from build123d import *

# Parameters (mm, degrees)
F0_R     = 5
F1_DEPTH = 10


with BuildPart() as f1:
    # F0 (on Right) → F1 (new body)
    with BuildSketch(Plane.YZ):
        Polygon((223.333333, 94.888889), (223.333333, 194.888889), (-196.666667, 194.888889), (-196.666667, -355.111111), (-96.666667, -355.111111), (-96.666667, 94.888889), align=None)
        with Locations((-116.666667, 144.888889)):
            Circle(F0_R, mode=Mode.SUBTRACT)
        with Locations((183.333333, 144.888889)):
            Circle(F0_R, mode=Mode.SUBTRACT)
    extrude(amount=F1_DEPTH)


solid = f1.part
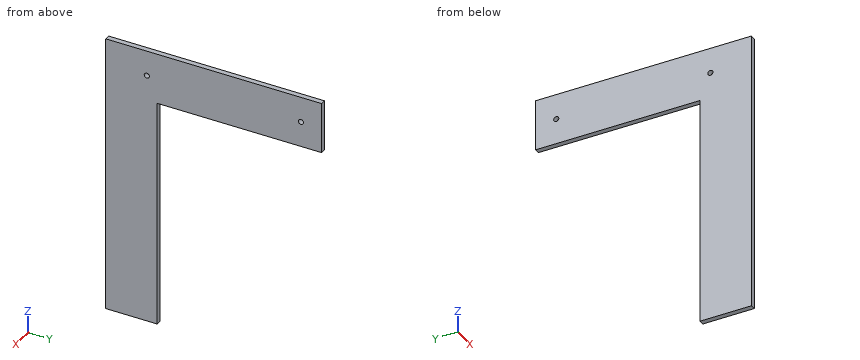
Geometry check sheet. Reference: the model listing, model coordinates, mm. Coordinates: 2 decimals unless noted, no trailing zeros. Order: outer loops, then holes, each group sorted by start corner. A loop starts at its lowest first (then second) coordinate and runs counter-clockwise, first axis right, second up. Notation, with made-up numbers: (-11.75, 16) -> (42.25, 16) arc R29 ccw to (42.25, 52) -> close; hole circle Ø1 at (75.5, -5). An arc over 180 degrees is marked (long way). Use a Markdown table: item, result. Add a question column.
1. Material ranges on L1, parallel to Y at x = 2, z = -186; L2, parallel to Z at x = 8.5, y = 73; L3, parallel to Z at x = 3.25, y = 184, recorded low to high.
2. Go/stop test with flat-tipped pins: pin 1 Ø2 at (x, y) = (2.5, 114) entering from -Z; pin 2 Ø1 at (y, z) = (-97.5, 44) entering from -X; pin 3 Ø9 at (y, z) = (183.33, 144.89) entering from +X; pin 4 Ø5 at (x, z) = (4.5, -128.5) entering from +Y. Record where each tip stops, or that it passes through.
3. Cross-section at B-B (z = -237). Enter the section's corners in (x, y).
4. Cross-section at C-C (y = 76.5). Enter the section's corners in (x, z), and give its area (3 significant figures).
5. Cross-section at A-A (x = 1.5). Enter the section's corners in (y, z).
Filled sheet:
| question | item | result |
|---|---|---|
| 1 | L1 | -196.67 to -96.67 |
| 1 | L2 | 94.89 to 194.89 |
| 1 | L3 | 94.89 to 139.93, 149.84 to 194.89 |
| 2 | pin 1 | z = 94.89 |
| 2 | pin 2 | x = 0 |
| 2 | pin 3 | through |
| 2 | pin 4 | y = -96.67 |
| 3 | outline | (0, -196.67) -> (10, -196.67) -> (10, -96.67) -> (0, -96.67) -> close |
| 4 | outline | (0, 94.89) -> (10, 94.89) -> (10, 194.89) -> (0, 194.89) -> close |
| 4 | area | 1,000 mm2 |
| 5 | outline | (-196.67, -355.11) -> (-96.67, -355.11) -> (-96.67, 94.89) -> (223.33, 94.89) -> (223.33, 194.89) -> (-196.67, 194.89) -> close; hole circle Ø10 at (-116.67, 144.89); hole circle Ø10 at (183.33, 144.89) |
